The model under review builds one solid part; all positions refer to its coordinate system, in mm. Face numbers are marked on the shaded views. A direction names the side the tool comes from. Coordinates: 2 decimals unless noted, no trailing zeros. Order: outer loops, then holes, each group sorted by start corner. A loop starts at its lowest first (then second) coordinate and runs counter-clockwise, first axis right, second up. Notation, with made-up numbers: M 31,-31.5 L 89,-31.5 A29 cw 89,-9.5 Z; hole C 34,11.25 d6. An arc over 180 degrees is marked long. Answer in a Markdown table with one row per item.
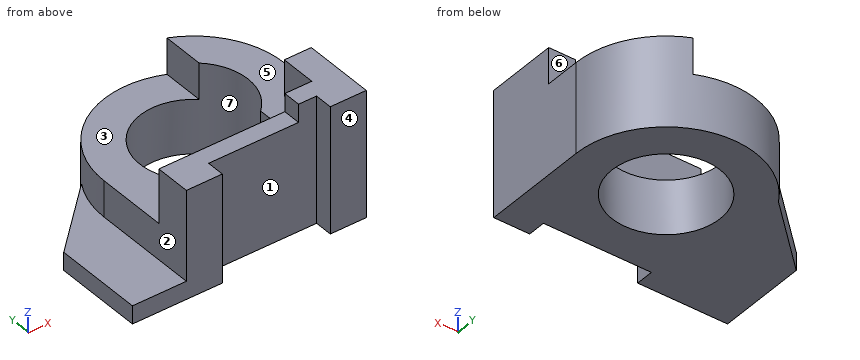
from build123d import *

# Parameters (mm, degrees)
SKETCH1_R           = 3
BOSS_EXTRUDE1_DEPTH = 7
BOSS_EXTRUDE2_DEPTH = 1
CUT_EXTRUDE1_DEPTH  = 2
CUT_EXTRUDE2_DEPTH  = 12
CUT_EXTRUDE3_DEPTH  = 12


with BuildPart() as part:
    # Sketch1 → Boss-Extrude1 (new body)
    with BuildSketch(Plane.XY):
        with BuildLine():
            Line((0, 0), (2, 0))
            Line((2, 0), (2, 1))
            Line((2, 1), (8, 1))
            Line((8, 1), (8, 0))
            Line((8, 0), (10, 0))
            Line((10, 0), (10, 6))
            ThreePointArc((10, 6), (5, 11), (0, 6))
            Line((0, 6), (0, 0))
        make_face()
        with Locations((5, 6)):
            Circle(SKETCH1_R, mode=Mode.SUBTRACT)
    extrude(amount=BOSS_EXTRUDE1_DEPTH)

    # Sketch2 → Boss-Extrude2 (add)
    with BuildSketch(Plane(origin=(0, 0, 0), x_dir=(-1, 0, 0), z_dir=(0, 0, -1))):
        Polygon((0, 0), (3, 0), (3, 5), (-0.705752773, 8.561140517), (-0.311985877, 0), align=None)
    extrude(amount=-BOSS_EXTRUDE2_DEPTH)

    # Sketch3 → Cut-Extrude1 (cut)
    with BuildSketch(Plane.XY.offset(7)):
        Polygon((7, 10.582575695), (7, 2), (8.5, 2), (8.5, 4), (10, 4), (10, 10.582575695), align=None)
    extrude(amount=-CUT_EXTRUDE1_DEPTH, mode=Mode.SUBTRACT)

    # Sketch4 → Cut-Extrude2 (cut)
    with BuildSketch(Plane(origin=(0, 0, 0), x_dir=(1, 0, 0), z_dir=(0, 1, 0))):
        Polygon((7, -7), (7, -6), (0, -6), (-0.727181491, -7.463826734), (7.362536443, -7.463826734), align=None)
    extrude(amount=CUT_EXTRUDE2_DEPTH, mode=Mode.SUBTRACT)

    # Sketch5 → Cut-Extrude3 (cut)
    with BuildSketch(Plane(origin=(0, 2, 0), x_dir=(1, 0, 0), z_dir=(0, 1, 0))):
        Polygon((7, -5), (7, -3), (0, -3), (0, -6), (7, -6), align=None)
    extrude(amount=CUT_EXTRUDE3_DEPTH, mode=Mode.SUBTRACT)


solid = part.part
(1) Take a section at C-C (y = 3.5). Write out the cut boundary in (x, z).
Report:
| item | result |
|---|---|
| outline | M -3,0 L 3.34,0 L 3.34,3 L 0,3 L 0,1 L -3,1 Z; M 6.66,0 L 10,0 L 10,7 L 8.5,7 L 8.5,5 L 7,5 L 7,3 L 6.66,3 Z |
(2) Insertion check: P1, Ø2, axis at x = 2, y = 6, coming from the +Z side; P2, Ø0.9, axis at x = 9, y = 5, coming from the +Z side; P3, Ø1.5, axis at x = 2, y = 2.5, coming from the +Z side. Each pin has a flat end and moves straight along its axis. Give the tip position at first contact, or say it passes through.
Report:
| item | result |
|---|---|
| P1 | z = 3 |
| P2 | z = 5 |
| P3 | z = 6 |
(3) The part is to be moulded in two halves that separate along Y. For the marked faces 4, 5, 6 and 7, say which applies: +Y half, -Y half, draft (parallel to the pull), parting line (faces both ways), or undercut.
Report:
| item | result |
|---|---|
| face 4 | -Y half |
| face 5 | draft |
| face 6 | +Y half |
| face 7 | undercut |
(4) Take a section at B-B (z = 2.25). Write out the cut boundary in (x, y), then the cut area to 3 significant figures.
Report:
| item | result |
|---|---|
| outline | M 0,0 L 2,0 L 2,1 L 8,1 L 8,0 L 10,0 L 10,6 A5 ccw 0,6 Z; hole C 5,6 d6 |
| area | 65.0 mm^2 |
(5) To check wall thickness, follow line 1 (Y direction, x = 5, z = 1.55); line 2 (Z direction, x = 2, y = 9); line 3 (Z direction, x = -2.5, y = 1.5). State the ranges of each line that lie inside material, in increasing order. Write a range as [from, to].
Report:
| item | result |
|---|---|
| line 1 | [1, 3], [9, 11] |
| line 2 | [0, 3] |
| line 3 | [0, 1] |
(6) Take a section at A-A (x = 5). Write out the cut boundary in (y, z), then the cut area to 3 significant figures.
Report:
| item | result |
|---|---|
| outline | M 1,0 L 3,0 L 3,3 L 2,3 L 2,6 L 1,6 Z; M 9,0 L 11,0 L 11,3 L 9,3 Z |
| area | 15.0 mm^2 |
(7) Take a section at D-D (z = 5.5). Write out the cut boundary in (x, y), then the cut area to 3 significant figures.
Report:
| item | result |
|---|---|
| outline | M 0,0 L 2,0 L 2,1 L 8,1 L 8,0 L 10,0 L 10,4 L 8.5,4 L 8.5,2 L 0,2 Z |
| area | 17.0 mm^2 |
(8) Machinability: for the marked faces 1, 2 and 3, which of the approach directions +Z, -Z, +X, -X, +Y, -Y give a long, thin tool a straight path to every point of the face, cutting with its end or side? Answer none if there is none.
Report:
| item | result |
|---|---|
| face 1 | +Z, -Z, -Y |
| face 2 | +Z, -X, +Y, -Y |
| face 3 | +Z, -X, +Y |
